```python
from build123d import *

# Parameters (mm, degrees)
SKETCH_1_W      = 70
SKETCH_1_H      = 53
EXTRUDE_1_DEPTH = 2
EXTRUDE_START   = 3
SKETCH_2_R      = 0.5
EXTRUDE_2_DEPTH = 48
SKETCH_3_R      = 0.5
EXTRUDE_3_DEPTH = 2.5


with BuildPart() as part:
    # Эскиз1 → Бобышка-Вытянуть1 (new body)
    with BuildSketch(Plane(origin=(0, 0, 0), x_dir=(0, 0, -1), z_dir=(1, 0, 0))):
        with Locations((0, 26.5)):
            Rectangle(SKETCH_1_W, SKETCH_1_H)
    extrude(amount=EXTRUDE_1_DEPTH)

    # Эскиз2 → Бобышка-Вытянуть2 (add)
    with BuildSketch(Plane(origin=(0, 0, 0), x_dir=(1, 0, 0), z_dir=(0, 1, 0)).offset(EXTRUDE_START)):
        with BuildLine():
            Line((2, 35), (3, 35))
            ThreePointArc((3, 35), (4, 34), (3, 33))
            Line((3, 33), (2, 33))
            Line((2, 33), (2, 35))
        make_face()
        with Locations(Location((3, 34, 0), (0, 0, 270))):
            Circle(SKETCH_2_R, mode=Mode.SUBTRACT)
    extrude_2 = extrude(amount=EXTRUDE_2_DEPTH)

    # Зеркальное отражение1: Бобышка-Вытянуть2 across plane
    add(extrude_2.mirror(Plane.XY))

    # Эскиз3 → Бобышка-Вытянуть3 (add, symmetric)
    with BuildSketch(Plane.XY):
        with BuildLine():
            Line((-1, 29), (0, 29))
            Line((0, 29), (0, 27))
            Line((0, 27), (-1, 27))
            ThreePointArc((-1, 27), (-2, 28), (-1, 29))
        make_face()
        with Locations((-1, 28)):
            Circle(SKETCH_3_R, mode=Mode.SUBTRACT)
    extrude(amount=EXTRUDE_3_DEPTH, both=True)


solid = part.part
```
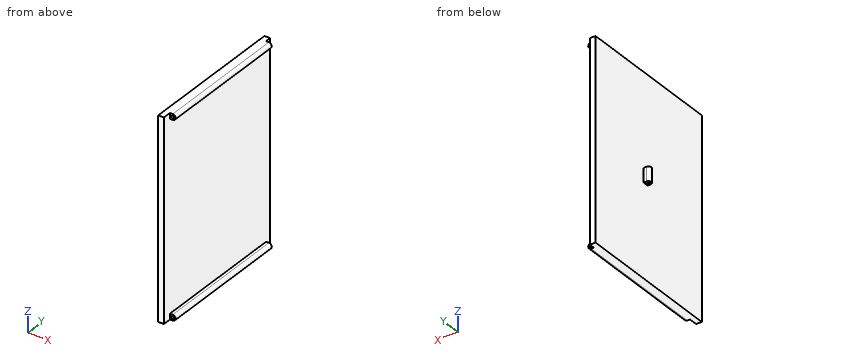
The listing builds one solid part. Answer for the finished solid, in the listing's coordinates (mm). Give positions to 0.01 mm unless a question says otherwise; leave off trailing zeros. Order: outer loops, then holes, each group sorted by start corner. A loop starts at its lowest first (then second) coordinate and runs counter-clockwise, first axis right, second up. Notation, with made-up numbers: (53, -33) -> (66, -33) arc R7 ccw to (66, -21) -> close; hole circle Ø7 at (-12.75, -29). An arc over 180 degrees is marked (long way). Write each question's results on one line, items separated by ' | '.
Q1. The part is cut by section A-A, the plane y = 42. Give the vertices of the cut face in (x, z).
Checked values:
outline: (0, -35) -> (3, -35) arc R1 ccw to (3, -33) -> (2, -33) -> (2, 33) -> (3, 33) arc R1 ccw to (3, 35) -> (0, 35) -> close; hole circle Ø1 at (3, -34); hole circle Ø1 at (3, 34)
Q2. Each of these flat-tipped pins is pushed along its axis until it touches: P1, Ø2, axis at y = 11.5, z = -9.5, coming from the -X side; P2, Ø2, axis at x = 3.5, z = 33.5, coming from the -Y side; P3, Ø2, axis at y = 44.5, z = 3.5, coming from the +X side; P4, Ø2, axis at x = 2.5, z = -34, coming from the +Y side. Where does it stop, or does it pass through?
Checked values:
P1: stops at x = 0 | P2: stops at y = 3 | P3: stops at x = 2 | P4: stops at y = 53
Q3. The part is cut by section B-B, the plane z = 25.5. Give the vertices of the cut face in (x, y).
Checked values:
outline: (0, 0) -> (2, 0) -> (2, 53) -> (0, 53) -> close
Q4. Straight lines are drawn through the part: probe 1 along Y at (x, z) = (-1, -1); probe 2 along Z at (x, y) = (3.1, 39); probe 3 along Z at (x, y) = (3.4, 29). For each, find the intervals that lie inside material, in ascending order. Write a range as from..to.
Checked values:
probe 1: y = 27..27.5, 28.5..29 | probe 2: z = -34.99..-34.49, -33.51..-33.01, 33.01..33.51, 34.49..34.99 | probe 3: z = -34.92..-34.3, -33.7..-33.08, 33.08..33.7, 34.3..34.92
